CAD build for the part. Positions are in the model's coordinates, mm. Face numbers are marked on the shaded views. A direction names the side the tool comes from. Coordinates: 2 decimals unless noted, no trailing zeros. Loops run counter-clockwise (first coordinate to the right, second up) from the corner with the lowest first, then second, coordinate; pieces in that order, holes last. Notation, with made-up numbers: (-33.75, 81.5) -> (-17.75, 81.5) arc R14 ccw to (-17.75, 98.5) -> close; hole circle Ø7 at (14, 58.5). An arc over 180 degrees is marked (long way). Return JSON: item names as keys, results as strings. Group by question number.
(1) Mould opens along Z. For the marked faces 3, 4 and 5 say: pulls with the +Z half, pulls with the -Z half, needs draft (parallel to the pull), parting line crosses it, or undercut.
(2) Saw through at D-D on y = 59.5. Write the cut outline in (x, z), then the cut area to 3 significant figures.
(3) Saw through at A-A on x = 0. Write the cut outline in (y, z), then the cut area to 3 significant figures.
(4) Probe L1, parallel to X at y = 55, z = 0; L2, parallel to Z at x = -27, y = -10.5; L3, parallel to Y at x = 4, z = -2. List the from-to ranges inside material, lowest first.
(5) Flat gauge pins, fed straight in: pin 1 Ø3.5 at (y, z) = (43, -8.5) entering from -X; pin 2 Ø0.9 at (y, z) = (57, -8.5) entering from +X; pin 3 Ø8.5 at (x, z) = (0, -31.18) entering from +Y. Where does each tip first touch, or does it go through?
(6) Saw through at B-B on y = -3. Give the number of separate pieces and of enclosed holes in the cut face, then the cut area to 3 significant figures.
(7) Tool access for the marked faces 1 and 2: list every direction of +Z, -Z, +X, -X, +Y, -Y with a clear straight run to the whole face (end or side of a thin tool).
(8) Saw through at C-C on z = 20. Write the cut outline in (x, y), then the cut area to 3 significant figures.
```python
from build123d import *

# Parameters (mm, degrees)
SKETCH1_R           = 25.34
BOSS_EXTRUDE1_DEPTH = 8.5
SKETCH2_R           = 25.34
BOSS_EXTRUDE2_DEPTH = 57.15
SKETCH7_R           = 25.34
BOSS_EXTRUDE4_DEPTH = 15
CUT_EXTRUDE3_DEPTH  = 115
SKETCH6_R           = 38.1
BOSS_EXTRUDE3_DEPTH = 15
CUT_EXTRUDE4_DEPTH  = 20
SKETCH10_R          = 2.75
CUT_EXTRUDE6_DEPTH  = 129
BOSS_EXTRUDE5_START = -93
BOSS_EXTRUDE5_DEPTH = 93
CUT_EXTRUDE8_START  = -10
SKETCH12_R          = 25.34
CUT_EXTRUDE8_DEPTH  = 10
SKETCH13_R          = 7.12
CUT_EXTRUDE9_DEPTH  = 40


with BuildPart() as part:
    # Sketch1 → Boss-Extrude1 (new body)
    with BuildSketch(Plane(origin=(0, 0, 0), x_dir=(1, 0, 0), z_dir=(0, 1, 0))):
        with Locations(Location((0, 0, 0), (0, 0, 270))):
            Circle(SKETCH1_R)
    extrude(amount=BOSS_EXTRUDE1_DEPTH)

    # Sketch2 → Boss-Extrude2 (add)
    with BuildSketch(Plane(origin=(0, 8.5, 0), x_dir=(1, 0, 0), z_dir=(0, 1, 0))):
        with Locations(Location((0, 0, 0), (0, 0, 270))):
            Circle(SKETCH2_R)
    extrude(amount=BOSS_EXTRUDE2_DEPTH)

    # Sketch7 → Boss-Extrude4 (add)
    with BuildSketch(Plane(origin=(0, 65.65, 0), x_dir=(1, 0, 0), z_dir=(0, 1, 0))):
        with Locations(Location((0, 0, 0), (0, 0, 270))):
            Circle(SKETCH7_R)
    extrude(amount=BOSS_EXTRUDE4_DEPTH)

    # Sketch5 → Cut-Extrude3 (cut)
    with BuildSketch(Plane.XZ):
        with BuildLine():
            ThreePointArc((2.575, 6.777305881), (0, 7.25), (-2.575, 6.777305881))
            Line((-2.575, 6.777305881), (-2.575, 4))
            Line((-2.575, 4), (2.575, 4))
            Line((2.575, 4), (2.575, 6.777305881))
        make_face()
        with BuildLine():
            Line((-2.575, 4), (-2.575, 6.777305881))
            ThreePointArc((-2.575, 6.777305881), (-4.116658232, -5.96788279), (7.25, 0))
            ThreePointArc((7.25, 0), (5.96788279, 4.116658232), (2.575, 6.777305881))
            Line((2.575, 6.777305881), (2.575, 4))
            Line((2.575, 4), (-2.575, 4))
        make_face()
        with BuildLine():
            Line((2.575, 9.15), (-2.575, 9.15))
            Line((-2.575, 9.15), (-2.575, 6.777305881))
            ThreePointArc((-2.575, 6.777305881), (0, 7.25), (2.575, 6.777305881))
            Line((2.575, 6.777305881), (2.575, 9.15))
        make_face()
    extrude(amount=-CUT_EXTRUDE3_DEPTH, mode=Mode.SUBTRACT)

    # Sketch6 → Boss-Extrude3 (add)
    with BuildSketch(Plane.XZ):
        with Locations(Location((0, 0, 0), (0, 0, 270))):
            Circle(SKETCH6_R)
    extrude(amount=BOSS_EXTRUDE3_DEPTH)

    # Sketch9 → Cut-Extrude4 (cut)
    with BuildSketch(Plane(origin=(0, 0, 0), x_dir=(1, 0, 0), z_dir=(0, 1, 0))):
        with BuildLine():
            ThreePointArc((-23.75, 15.588457268), (-23.860741065, 16.429619165), (-24.185417438, 17.213457268))
            Line((-24.185417438, 17.213457268), (-27, 15.588457268))
            Line((-27, 15.588457268), (-27, 12.338457268))
            ThreePointArc((-27, 12.338457268), (-24.701902961, 13.290360229), (-23.75, 15.588457268))
        make_face()
        with BuildLine():
            Line((-27, 15.588457268), (-24.185417438, 17.213457268))
            ThreePointArc((-24.185417438, 17.213457268), (-29.814582562, 17.213457268), (-27, 12.338457268))
            Line((-27, 12.338457268), (-27, 15.588457268))
        make_face()
        with BuildLine():
            Line((2.814582562, 29.551914536), (0, 31.176914536))
            Line((0, 31.176914536), (-2.814582562, 29.551914536))
            ThreePointArc((-2.814582562, 29.551914536), (0, 27.926914536), (2.814582562, 29.551914536))
        make_face()
        with BuildLine():
            Line((-2.814582562, 29.551914536), (0, 31.176914536))
            Line((0, 31.176914536), (2.814582562, 29.551914536))
            ThreePointArc((2.814582562, 29.551914536), (3.139258935, 30.33575264), (3.25, 31.176914536))
            ThreePointArc((3.25, 31.176914536), (-0.841161897, 34.316173472), (-2.814582562, 29.551914536))
        make_face()
        with BuildLine():
            ThreePointArc((30.25, 15.588457268), (27.841161897, 18.727716204), (24.185417438, 17.213457268))
            Line((24.185417438, 17.213457268), (27, 15.588457268))
            Line((27, 15.588457268), (27, 12.338457268))
            ThreePointArc((27, 12.338457268), (29.298097039, 13.290360229), (30.25, 15.588457268))
        make_face()
        with BuildLine():
            Line((27, 15.588457268), (24.185417438, 17.213457268))
            ThreePointArc((24.185417438, 17.213457268), (24.185417438, 13.963457268), (27, 12.338457268))
            Line((27, 12.338457268), (27, 15.588457268))
        make_face()
        with BuildLine():
            ThreePointArc((30.25, -15.588457268), (29.298097039, -13.290360229), (27, -12.338457268))
            Line((27, -12.338457268), (27, -15.588457268))
            Line((27, -15.588457268), (24.185417438, -17.213457268))
            ThreePointArc((24.185417438, -17.213457268), (27.841161897, -18.727716204), (30.25, -15.588457268))
        make_face()
        with BuildLine():
            Line((27, -15.588457268), (27, -12.338457268))
            ThreePointArc((27, -12.338457268), (24.185417438, -13.963457268), (24.185417438, -17.213457268))
            Line((24.185417438, -17.213457268), (27, -15.588457268))
        make_face()
        with BuildLine():
            ThreePointArc((2.814582562, -29.551914536), (0, -27.926914536), (-2.814582562, -29.551914536))
            Line((-2.814582562, -29.551914536), (0, -31.176914536))
            Line((0, -31.176914536), (2.814582562, -29.551914536))
        make_face()
        with BuildLine():
            Line((0, -31.176914536), (-2.814582562, -29.551914536))
            ThreePointArc((-2.814582562, -29.551914536), (-0.841161897, -34.316173472), (3.25, -31.176914536))
            ThreePointArc((3.25, -31.176914536), (3.139258935, -30.33575264), (2.814582562, -29.551914536))
            Line((2.814582562, -29.551914536), (0, -31.176914536))
        make_face()
        with BuildLine():
            ThreePointArc((-23.75, -15.588457268), (-24.701902961, -13.290360229), (-27, -12.338457268))
            Line((-27, -12.338457268), (-27, -15.588457268))
            Line((-27, -15.588457268), (-24.185417438, -17.213457268))
            ThreePointArc((-24.185417438, -17.213457268), (-23.860741065, -16.429619165), (-23.75, -15.588457268))
        make_face()
        with BuildLine():
            Line((-27, -15.588457268), (-27, -12.338457268))
            ThreePointArc((-27, -12.338457268), (-29.814582562, -17.213457268), (-24.185417438, -17.213457268))
            Line((-24.185417438, -17.213457268), (-27, -15.588457268))
        make_face()
    extrude(amount=-CUT_EXTRUDE4_DEPTH, mode=Mode.SUBTRACT)

    # Sketch10 → Cut-Extrude6 (cut)
    with BuildSketch(Plane(origin=(0, 80.65, 0), x_dir=(1, 0, 0), z_dir=(0, 1, 0))):
        with Locations(Location((0, 20, 0), (0, 0, 270))):
            Circle(SKETCH10_R)
        with Locations(Location((0, -20, 0), (0, 0, 270))):
            Circle(SKETCH10_R)
    extrude(amount=-CUT_EXTRUDE6_DEPTH, mode=Mode.SUBTRACT)

    # Sketch11 → Boss-Extrude5 (add)
    with BuildSketch(Plane(origin=(0, 80.65, 0), x_dir=(1, 0, 0), z_dir=(0, 1, 0)).offset(BOSS_EXTRUDE5_START)):
        with BuildLine():
            Line((-2.575, -6.777305881), (-2.575, -9.15))
            Line((-2.575, -9.15), (0, -9.15))
            Line((0, -9.15), (2.575, -9.15))
            Line((2.575, -9.15), (2.575, -6.777305881))
            ThreePointArc((2.575, -6.777305881), (0, 7.25), (-2.575, -6.777305881))
        make_face()
    extrude(amount=BOSS_EXTRUDE5_DEPTH)

    # Sketch12 → Cut-Extrude8 (cut)
    with BuildSketch(Plane(origin=(0, 80.65, 0), x_dir=(1, 0, 0), z_dir=(0, 1, 0)).offset(CUT_EXTRUDE8_START)):
        with Locations(Location((0, 0, 0), (0, 0, 270))):
            Circle(SKETCH12_R)
    extrude(amount=CUT_EXTRUDE8_DEPTH, mode=Mode.SUBTRACT)

    # Sketch13 → Cut-Extrude9 (cut)
    with BuildSketch(Plane(origin=(0, 70.65, 0), x_dir=(1, 0, 0), z_dir=(0, 1, 0))):
        Polygon((2.51482759, 9.62638963), (2.51482759, 7.12), (0, 7.12), (-2.51482759, 7.12), (-2.51482759, 9.62638963), align=None)
        Circle(SKETCH13_R)
        with BuildLine():
            ThreePointArc((-2.51482759, 6.66108416), (-1.278178543, 7.004331489), (0, 7.12))
            Line((0, 7.12), (-2.51482759, 7.12))
            Line((-2.51482759, 7.12), (-2.51482759, 6.66108416))
        make_face()
        with BuildLine():
            Line((2.51482759, 7.12), (0, 7.12))
            ThreePointArc((0, 7.12), (1.278178543, 7.004331489), (2.51482759, 6.66108416))
            Line((2.51482759, 6.66108416), (2.51482759, 7.12))
        make_face()
    extrude(amount=-CUT_EXTRUDE9_DEPTH, mode=Mode.SUBTRACT)


solid = part.part
```
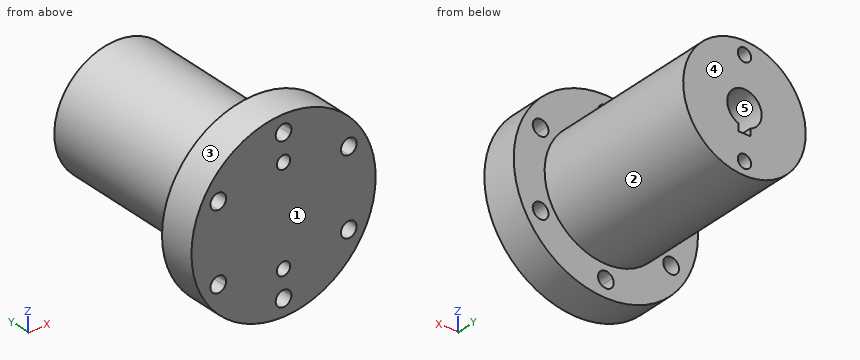
Geometry results:
{
 "1": {"face 3": "parting line crosses it", "face 4": "needs draft", "face 5": "undercut"},
 "2": {"outline": "circle Ø50.68 at (0, 0); hole circle Ø5.5 at (0, -20); hole circle Ø5.5 at (0, 20); hole (-2.51, -9.63) -> (2.51, -9.63) -> (2.51, -6.66) arc R7.12 ccw (long way) to (-2.51, -6.66) -> close", "area": "1,800 mm²"},
 "3": {"outline": "(-15, -38.1) -> (0, -38.1) -> (0, -34.43) -> (-15, -34.43) -> close; (-15, -27.93) -> (0, -27.93) -> (0, -25.34) -> (70.65, -25.34) -> (70.65, -22.75) -> (-15, -22.75) -> close; (-15, -17.25) -> (70.65, -17.25) -> (70.65, -9.63) -> (30.65, -9.63) -> (30.65, 7.12) -> (70.65, 7.12) -> (70.65, 17.25) -> (-15, 17.25) -> close; (-15, 22.75) -> (70.65, 22.75) -> (70.65, 25.34) -> (0, 25.34) -> (0, 27.93) -> (-15, 27.93) -> close; (-15, 34.43) -> (0, 34.43) -> (0, 38.1) -> (-15, 38.1) -> close", "area": "2,920 mm²"},
 "4": {"L1": "-25.34 to -7.12, 7.12 to 25.34", "L2": "-26.88 to -18.84, -12.34 to 12.34, 18.84 to 26.88", "L3": "-15 to 30.65"},
 "5": {"pin 1": "x = -24.42", "pin 2": "x = 24.03", "pin 3": "y = 0"},
 "6": {"separate pieces": "1", "enclosed holes": "8", "area": "4,310 mm²"},
 "7": {"face 1": "+Z, -Z, +X, -X, -Y", "face 2": "+Y"},
 "8": {"outline": "(-32.43, -15) -> (-2.75, -15) -> (-2.75, 70.65) -> (-15.56, 70.65) -> (-15.56, 0) -> (-32.43, 0) -> close; (2.75, -15) -> (32.43, -15) -> (32.43, 0) -> (15.56, 0) -> (15.56, 70.65) -> (2.75, 70.65) -> close", "area": "2,700 mm²"}
}
